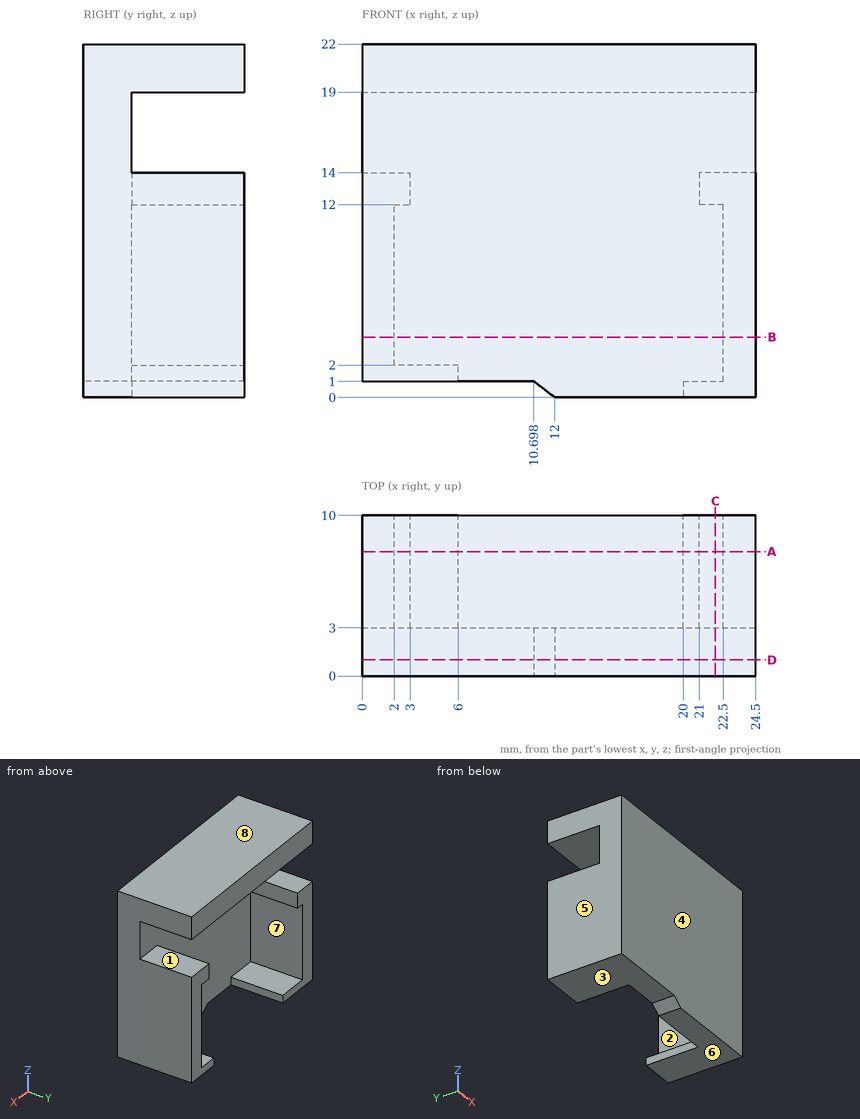
Input: dimensioned drawing with shaded views. Units: mm. Origin: part minimum x, y, z. A direction names the side the tool comes from. Coordinates: 2 decimals unless noted, no trailing zeros. Loops run counter-clockwise (first coordinate to the right, second up) from the corner with the lowest first, then second, coordinate; pieces in that order, holes last. Notation, with made-up numbers: M 10.25,42 L 21.25,42 A20 cw 21.25,53 Z; hole C 86,85.25 d9. An arc over 180 degrees is marked long. Use a Markdown table: item, result. Add a question column.
Q1. Section query C-C, the plane x = 22. Return loops of the section in (y, z).
Q2. Section query B-B, the plane z = 3.75. Return loops of the section in (x, y).
Q3. Access query for the marked faces 1, 2, 3 and 4. Directions: +Z, -Z, +X, -X, +Y, -Y. A direction counts if a zero-diameter tool reaches every point of the face in a straight line with its end or side. Return the directions, or none.
Q4. Draft query along Z for the marked faces 5, 6, 7 and 8. Return one class per face: pulls with the +Z half, pulls with the -Z half, needs draft (parallel to the pull), parting line crosses it, or undercut.
Q5. Material intervals for L1, parallel to Z at x = 23, y = 9; L2, parallel to X at y = 8.5, z = 13; L3, parallel to X at y = 9, z = 2.75, sorted ascending.
Q6. Section query D-D, the plane y = 1. Return loops of the section in (x, z), and give its area (3 significant figures).
Q7. Section query A-A, the plane y = 7.75. Return loops of the section in (x, z).
Q8. First-contact query: pin 1 (6 mm diameter, centred on x = 14.5, z = 2.5, fed in from +Y); pin 2 (0.5 mm diameter, centred on y = 8, z = 0.5, fed in from -X); pin 3 (3.5 mm diameter, centred on x = 8, y = 5.5, fed in from -Z). Flat tips, straight axial feed; report the tip coordinate or a pass-through.
Result:
| question | item | result |
|---|---|---|
| 1 | outline | M 0,0 L 10,0 L 10,1 L 3,1 L 3,12 L 10,12 L 10,14 L 3,14 L 3,19 L 10,19 L 10,22 L 0,22 Z |
| 2 | outline | M 0,0 L 24.5,0 L 24.5,10 L 22.5,10 L 22.5,3 L 2,3 L 2,10 L 0,10 Z |
| 3 | face 1 | +X, -X, +Y |
| 3 | face 2 | +Y |
| 3 | face 3 | -Z, -X, +Y, -Y |
| 3 | face 4 | +Z, -Z, +X, -X, -Y |
| 4 | face 5 | needs draft |
| 4 | face 6 | pulls with the -Z half |
| 4 | face 7 | undercut |
| 4 | face 8 | pulls with the +Z half |
| 5 | L1 | z = 0 to 14, 19 to 22 |
| 5 | L2 | x = 0 to 3, 21 to 24.5 |
| 5 | L3 | x = 0 to 2, 22.5 to 24.5 |
| 6 | outline | M 0,1 L 10.7,1 L 12,0 L 24.5,0 L 24.5,22 L 0,22 Z |
| 6 | area | 528 mm2 |
| 7 | outline | M 0,1 L 6,1 L 6,2 L 2,2 L 2,12 L 3,12 L 3,14 L 0,14 Z; M 0,19 L 24.5,19 L 24.5,22 L 0,22 Z; M 20,0 L 24.5,0 L 24.5,14 L 21,14 L 21,12 L 22.5,12 L 22.5,1 L 20,1 Z |
| 8 | pin 1 | stops at y = 3 |
| 8 | pin 2 | stops at x = 20 |
| 8 | pin 3 | stops at z = 19 |
